Can you work these out from the model? Positions are in its coordinate system, mm. Round coordinates to 2 decimals unless told otherwise and drop trailing zeros. Write item = value, one per line.
from build123d import *

# Parameters (mm, degrees)
F1_DEPTH = 5


with BuildPart() as f1:
    # F0 (on Front) → F1 (new body)
    with BuildSketch(Plane.XZ):
        Polygon((98.954107, -74.362564), (104.19903, -77.978152), (109.668386, -81.244313), (115.338936, -84.147177), (121.18655, -86.674401), (127.186436, -88.81524), (133.313043, -90.560601), (183.300167, -89.426237), (179.215694, 90.560601), (110.167471, 88.993675), (105.265372, 88.715596), (100.393449, 88.10531), (95.574231, 87.165612), (90.829917, 85.900844), (86.182454, 84.316849), (81.653253, 82.420968), (77.263269, 80.221912), (73.032696, 77.729842), (68.981142, 74.956264), (65.127251, 71.913979), (61.488803, 68.617033), (58.082663, 65.080642), (47.36272, 53.16601), (40.946045, 46.278343), (34.294343, 39.617396), (27.415617, 33.191171), (20.31812, 27.007388), (13.010413, 21.073491), (5.501284, 15.396642), (-2.200199, 9.983673), (-10.084816, 4.841088), (-18.143068, -0.024943), (-26.365251, -4.608551), (-34.74146, -8.904199), (-43.26161, -12.906756), (133.402603, -22.155506), (133.854063, -28.785007), (108.662673, -29.356685), (108.617309, -27.357197), (68.6276, -28.264688), (68.672964, -30.264176), (13.68712, -31.511977), (-183.300167, -35.98225), (-181.325495, -40.492528), (-179.012799, -44.839153), (-176.375517, -48.996879), (-173.429016, -52.941474), (-170.190414, -56.650001), (-166.678559, -60.100921), (-162.913898, -63.274092), (-158.9183, -66.1511), (-154.715058, -68.715204), (-150.328605, -70.951446), (-145.784468, -72.846844), (-141.109065, -74.390402), (-135.176895, -75.819813), (-129.14155, -76.719024), (-123.050325, -77.080999), (-116.950947, -76.90292), (-110.891218, -76.186132), (-104.918612, -74.936274), (-99.079939, -73.163151), (-93.420946, -70.880656), (-87.985981, -68.106646), (-82.817589, -64.862913), (-77.956334, -61.174808), (-73.440239, -57.07126), (-60.687026, -52.802841), (-47.687916, -49.355121), (-34.495664, -46.742045), (-21.163813, -44.974281), (-7.746441, -44.058942), (5.701995, -43.999785), (19.126911, -44.79704), (32.473798, -46.447456), (45.688529, -48.944352), (58.717485, -52.277594), (71.507756, -56.433644), (73.871785, -57.805904), (76.22253, -59.200745), (78.559838, -60.618065), (80.88343, -62.057712), (83.193128, -63.519558), (85.488729, -65.003451), (87.769979, -66.50929), (90.036701, -68.036923), (92.28869, -69.586221), (94.525719, -71.157008), (96.747584, -72.749181), align=None)
    extrude(amount=F1_DEPTH)


solid = f1.part
1. I'm going to push flat-ended pins straight in: pin 1 (3 mm diameter, centred on y = -3.5, z = -42, fed in from +X); pin 2 (1.5 mm diameter, centred on y = -2, z = 53, fed in from -X); pin 3 (3 mm diameter, centred on y = -4, z = 68.5, fed in from -X). Where does each tip first touch, or does it pass through?
Entries:
pin_1 = 182.26
pin_2 = 46.51
pin_3 = 59.93
2. I need wall thicknesses on line 1 (Z direction, x = -22, y = -2.2); line 2 (Z direction, x = 116, y = -0.8); line 3 (X direction, y = -1.5, z = -64.5). Which ranges of each line are inside material? Lowest first, please. Write a range as [from, to].
Entries:
line_1 = [-45.09, -32.32], [-14.02, -2.18]
line_2 = [-84.43, -29.19], [-21.24, 89.13]
line_3 = [-161.21, -82.34], [84.71, 182.73]
3. We'd pull the mould along Z, two halves only. Please class faces 1 (the flat face through (43.834, -2.465, -17.466)), 2 (the flat face through (79, 0, 1)), 3 (the flat face through (44.2, -2.46, 49.77)): released by +Z, released by -Z, zero draft, split by the parting line, or undercut.
Entries:
face_1 = undercut
face_2 = zero draft
face_3 = released by +Z
